Design review of the part built by this model. Coordinates are the model's own, in mm. Face numbers are marked on the shaded views. Coordinates: 2 decimals unless noted, no trailing zeros. Loops run counter-clockwise (first coordinate to the right, second up) from the corner with the lowest first, then second, coordinate; pieces in that order, holes last.
from build123d import *

# Parameters (mm, degrees)
BOSS_EXTRU_1_DEPTH      = 5
ENL_V_MAT_EXTRU_1_REACH = 129.849
ESQUISSE2_R             = 1.5
ENL_V_MAT_EXTRU_2_REACH = 136.797
ESQUISSE3_R             = 1.5
ENL_V_MAT_EXTRU_3_REACH = 129.849
ESQUISSE4_R             = 1.5
ENL_V_MAT_EXTRU_4_REACH = 129.615
ESQUISSE5_R             = 1.5
ESQUISSE6_R             = 3.5
ESQUISSE6_R_2           = 1.5
BOSS_EXTRU_2_DEPTH      = 30
ENL_V_MAT_EXTRU_5_REACH = 142.518
ESQUISSE7_R             = 1.5
ESQUISSE8_W             = 34
ESQUISSE8_H             = 25
ENL_V_MAT_EXTRU_6_DEPTH = 5
ESQUISSE9_W             = 51
ESQUISSE9_H             = 51
ENL_V_MAT_EXTRU_7_DEPTH = 2


with BuildPart() as part:
    # Esquisse1 → Boss.-Extru.1 (new body)
    with BuildSketch(Plane.XY):
        Polygon((15.5, 95.5), (15.5, 90.5), (5, 90.5), (5, 80), (0, 80), (0, 61), (5, 61), (5, 35), (0, 35), (0, 16), (5, 16), (5, 5.5), (15.5, 5.5), (15.5, 0.5), (34.5, 0.5), (34.5, 5.5), (65.5, 5.5), (65.5, 0.5), (84.5, 0.5), (84.5, 5.5), (95, 5.5), (95, 16), (100, 16), (100, 35), (95, 35), (95, 61), (100, 61), (100, 80), (95, 80), (95, 90.5), (84.5, 90.5), (84.5, 95.5), (65.5, 95.5), (65.5, 90.5), (34.5, 90.5), (34.5, 95.5), align=None)
    extrude(amount=BOSS_EXTRU_1_DEPTH)

    # Enlèv. mat.-Extru.1: up to this face of the body (flat: up to its plane)
    enl_v_mat_extru_1_end = Plane(part.part.faces().sort_by_distance((97.5, 80, 2.5))[0])
    # Esquisse2 → Enlèv. mat.-Extru.1 (cut, up to the picked face)
    with BuildSketch(Plane.XZ.offset(-16), mode=Mode.PRIVATE) as enl_v_mat_extru_1_sk1:
        with Locations((97.5, 2.5)):
            Circle(ESQUISSE2_R)
    enl_v_mat_extru_1_tool1 = split(extrude(enl_v_mat_extru_1_sk1.sketch, amount=-ENL_V_MAT_EXTRU_1_REACH, mode=Mode.PRIVATE), bisect_by=enl_v_mat_extru_1_end, keep=Keep.BOTH, mode=Mode.PRIVATE)
    add(enl_v_mat_extru_1_tool1.solids().sort_by(Axis((97.5, 16, 2.5), (0, 1, 0)))[0], mode=Mode.SUBTRACT)

    # Enlèv. mat.-Extru.2: up to this face of the body (flat: up to its plane)
    enl_v_mat_extru_2_end = Plane(part.part.faces().sort_by_distance((5, 85.25, 2.5))[0])
    # Esquisse3 → Enlèv. mat.-Extru.2 (cut, up to the picked face)
    with BuildSketch(Plane(origin=(95, 0, 0), x_dir=(0, 0, -1), z_dir=(1, 0, 0)), mode=Mode.PRIVATE) as enl_v_mat_extru_2_sk1:
        with Locations(Location((-2.5, 93, 0), (0, 0, 90))):
            Circle(ESQUISSE3_R)
    enl_v_mat_extru_2_tool1 = split(extrude(enl_v_mat_extru_2_sk1.sketch, amount=-ENL_V_MAT_EXTRU_2_REACH, mode=Mode.PRIVATE), bisect_by=enl_v_mat_extru_2_end, keep=Keep.BOTH, mode=Mode.PRIVATE)
    add(enl_v_mat_extru_2_tool1.solids().sort_by(Axis((95, 93, 2.5), (-1, 0, 0)))[0], mode=Mode.SUBTRACT)

    # Enlèv. mat.-Extru.3: up to this face of the body (flat: up to its plane)
    enl_v_mat_extru_3_end = Plane(part.part.faces().sort_by_distance((2.5, 16, 2.5))[0])
    # Esquisse4 → Enlèv. mat.-Extru.3 (cut, up to the picked face)
    with BuildSketch(Plane(origin=(0, 80, 0), x_dir=(1, 0, 0), z_dir=(0, 1, 0)), mode=Mode.PRIVATE) as enl_v_mat_extru_3_sk1:
        with Locations(Location((2.5, -2.5, 0), (0, 0, 270))):
            Circle(ESQUISSE4_R)
    enl_v_mat_extru_3_tool1 = split(extrude(enl_v_mat_extru_3_sk1.sketch, amount=-ENL_V_MAT_EXTRU_3_REACH, mode=Mode.PRIVATE), bisect_by=enl_v_mat_extru_3_end, keep=Keep.BOTH, mode=Mode.PRIVATE)
    add(enl_v_mat_extru_3_tool1.solids().sort_by(Axis((2.5, 80, 2.5), (0, -1, 0)))[0], mode=Mode.SUBTRACT)

    # Enlèv. mat.-Extru.4: up to this face of the body (flat: up to its plane)
    enl_v_mat_extru_4_end = Plane(part.part.faces().sort_by_distance((84.5, 3, 2.5))[0])
    # Esquisse5 → Enlèv. mat.-Extru.4 (cut, up to the picked face)
    with BuildSketch(Plane.ZY.offset(-15.5), mode=Mode.PRIVATE) as enl_v_mat_extru_4_sk1:
        with Locations((2.5, 3)):
            Circle(ESQUISSE5_R)
    enl_v_mat_extru_4_tool1 = split(extrude(enl_v_mat_extru_4_sk1.sketch, amount=-ENL_V_MAT_EXTRU_4_REACH, mode=Mode.PRIVATE), bisect_by=enl_v_mat_extru_4_end, keep=Keep.BOTH, mode=Mode.PRIVATE)
    add(enl_v_mat_extru_4_tool1.solids().sort_by(Axis((15.5, 3, 2.5), (1, 0, 0)))[0], mode=Mode.SUBTRACT)

    # Esquisse6 → Boss.-Extru.2 (add)
    with BuildSketch(Plane(origin=(0, 0, 0), x_dir=(-1, 0, 0), z_dir=(0, 0, -1))):
        with Locations((-31, 25.5)):
            Circle(ESQUISSE6_R)
        with Locations((-31, 25.5)):
            Circle(ESQUISSE6_R_2, mode=Mode.SUBTRACT)
    extrude(amount=-BOSS_EXTRU_2_DEPTH)

    # Esquisse7 → Enlèv. mat.-Extru.5 (cut, up to next)
    with BuildSketch(Plane.XY.offset(5), mode=Mode.PRIVATE) as enl_v_mat_extru_5_sk1:
        with Locations(Location((31, 25.5, 0), (0, 0, 180))):
            Circle(ESQUISSE7_R)
    enl_v_mat_extru_5_tool1 = extrude(enl_v_mat_extru_5_sk1.sketch, amount=-ENL_V_MAT_EXTRU_5_REACH, mode=Mode.PRIVATE) & part.part
    add(enl_v_mat_extru_5_tool1.solids().sort_by_distance((31, 25.5, 5))[0], mode=Mode.SUBTRACT)

    # Esquisse8 → Enlèv. mat.-Extru.6 (cut)
    with BuildSketch(Plane(origin=(0, 0, 0), x_dir=(-1, 0, 0), z_dir=(0, 0, -1))):
        with Locations((-74, 43)):
            Rectangle(ESQUISSE8_W, ESQUISSE8_H)
    extrude(amount=-ENL_V_MAT_EXTRU_6_DEPTH, mode=Mode.SUBTRACT)

    # Esquisse9 → Enlèv. mat.-Extru.7 (cut)
    with BuildSketch(Plane(origin=(0, 0, 0), x_dir=(-1, 0, 0), z_dir=(0, 0, -1))):
        with Locations((-65.5, 43)):
            Rectangle(ESQUISSE9_W, ESQUISSE9_H)
    extrude(amount=-ENL_V_MAT_EXTRU_7_DEPTH, mode=Mode.SUBTRACT)


solid = part.part
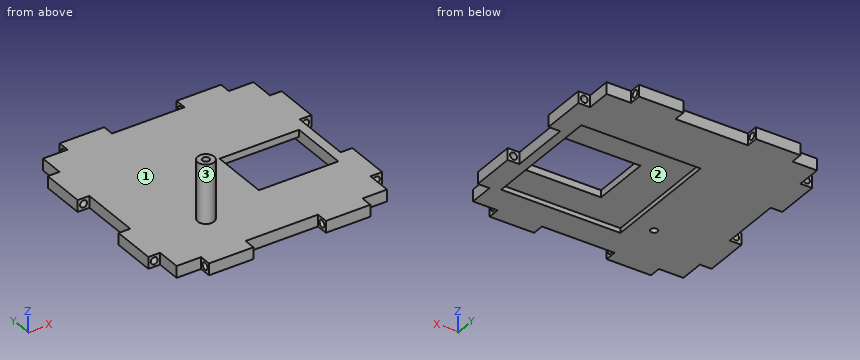
Q1. Take a section at A-A, the plane x = 80. Write out the cut boundary in (y, z).
Q2. Clearance check with flat-ended pins moving along their axes: pin 1 Ø1.5 at (y, z) = (3, 3.5) entering from -X; pin 2 Ø1 at (y, z) = (48, 1.5) entering from +X; pin 3 Ø3.5 at (y, z) = (3, 2.5) entering from +X; pin 4 Ø5 at (x, y) = (32.5, 15) entering from -Z. State where each tip first meets the part, or that it passes through.
Q3. Take a section at D-D, the plane x = 2.5. Write out the cut boundary in (y, z).
Q4. Take a section at C-C, the plane y = 25.5. Write out the cut boundary in (x, z).
Q5. The part is to be moulded in two halves that separate along X. For the marked faces 1, 2 and 3, say which applies: pulls with the +X half, pulls with the -X half, needs draft (parallel to the pull), parting line crosses it, or undercut.
Q6. For line 1 (Z direction, x = 24.75, y = 93); line 2 (Z direction, x = 94.5, y = 82.5); line 3 (Y direction, x = 73, z = 4.5), list the stretches that pass through material, from the lowest coordinate up.
Q7. Take a section at B-B, the plane y = 93. Write out the cut boundary in (x, z), then the cut area to 3 significant figures.
Entries:
1. outline: (0.5, 0) - (17.5, 0) - (17.5, 2) - (30.5, 2) - (30.5, 5) - (0.5, 5) - close; (55.5, 2) - (68.5, 2) - (68.5, 0) - (95.5, 0) - (95.5, 5) - (55.5, 5) - close; hole circle Ø3 at (3, 2.5); hole circle Ø3 at (93, 2.5)
2. pin 1: stops at x = 15.5
2. pin 2: stops at x = 95
2. pin 3: stops at x = 84.5
2. pin 4: stops at z = 0
3. outline: (16, 0) - (35, 0) - (35, 1) - (16, 1) - close; (16, 4) - (35, 4) - (35, 5) - (16, 5) - close; (61, 0) - (80, 0) - (80, 1) - (61, 1) - close; (61, 4) - (80, 4) - (80, 5) - (61, 5) - close
4. outline: (0, 0) - (29.5, 0) - (29.5, 30) - (27.5, 30) - (27.5, 5) - (0, 5) - close; (32.5, 0) - (40, 0) - (40, 2) - (91, 2) - (91, 0) - (100, 0) - (100, 5) - (34.5, 5) - (34.5, 30) - (32.5, 30) - close; hole circle Ø3 at (2.5, 2.5); hole circle Ø3 at (97.5, 2.5)
5. face 1: needs draft
5. face 2: undercut
5. face 3: parting line crosses it
6. line 1: z = 0 to 1, 4 to 5
6. line 2: z = 0 to 5
6. line 3: y = 0.5 to 30.5, 55.5 to 95.5
7. outline: (15.5, 0) - (34.5, 0) - (34.5, 1) - (15.5, 1) - close; (15.5, 4) - (34.5, 4) - (34.5, 5) - (15.5, 5) - close; (65.5, 0) - (84.5, 0) - (84.5, 1) - (65.5, 1) - close; (65.5, 4) - (84.5, 4) - (84.5, 5) - (65.5, 5) - close
7. area: 76.0 mm2
